Geometry: final body of the model. Coordinates: model frame, mm. Give positions to 0.01 mm unless a question says otherwise; leave off trailing zeros. Write each loop counter-clockwise with the first axis right and the second up, starting at its lowest first coordinate (ties: lowest second). Pieces come first, ordered by that corner, then holes. Notation, with made-up numbers: M 44.25,37 L 93.25,37 A37 cw 93.25,74 Z; hole C 33,30.5 d9. An arc over 180 degrees is marked long. Answer as a JSON object with one key per item and string values.
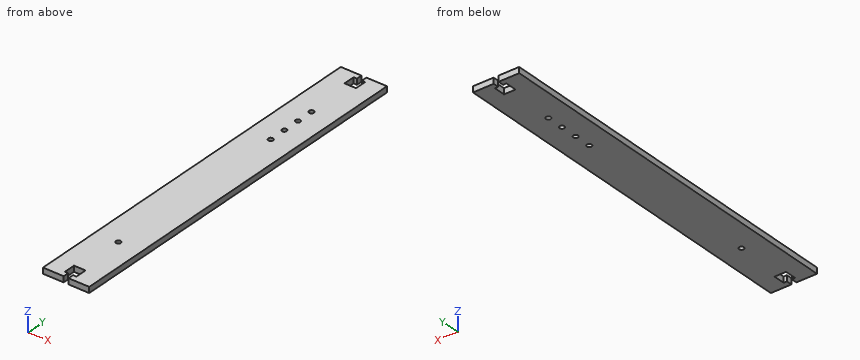
from build123d import *

# Parameters (mm, degrees)
SKETCH1_W           = 40
SKETCH1_H           = 327.5
BOSS_EXTRUDE1_DEPTH = 5
SKETCH2_R           = 2.1
CUT_EXTRUDE1_DEPTH  = 5
CUT_EXTRUDE2_DEPTH  = 5


with BuildPart() as part:
    # Sketch1 → Boss-Extrude1 (new body)
    with BuildSketch(Plane.XY):
        with Locations((-20, 163.75)):
            Rectangle(SKETCH1_W, SKETCH1_H)
    extrude(amount=BOSS_EXTRUDE1_DEPTH)

    # Sketch2 → Cut-Extrude1 (cut)
    with BuildSketch(Plane(origin=(0, 0, 0), x_dir=(-1, 0, 0), z_dir=(0, 0, -1))):
        with Locations((20, 57.5)):
            Circle(SKETCH2_R)
        with Locations((20, 270)):
            Circle(SKETCH2_R)
        with Locations((20, 255)):
            Circle(SKETCH2_R)
        with Locations((20, 240)):
            Circle(SKETCH2_R)
        with Locations((20, 225)):
            Circle(SKETCH2_R)
    extrude(amount=-CUT_EXTRUDE1_DEPTH, mode=Mode.SUBTRACT)

    # Sketch3 → Cut-Extrude2 (cut)
    with BuildSketch(Plane(origin=(0, 0, 0), x_dir=(-1, 0, 0), z_dir=(0, 0, -1))):
        Polygon((17.9, 0), (22.1, 0), (22.1, 5), (25, 5), (25, 15), (15, 15), (15, 5), (17.9, 5), align=None)
    cut_extrude2 = extrude(amount=-CUT_EXTRUDE2_DEPTH, mode=Mode.SUBTRACT)

    # Mirror1: Cut-Extrude2 across plane
    add(cut_extrude2.mirror(Plane.ZX.offset(163.75)), mode=Mode.SUBTRACT)


solid = part.part
1) Line query: line 1 (Y direction, x = -20, z = 1.2); line 2 (Y direction, x = -20.5, z = 4.3); line 3 (X direction, y = 225, z = 1.4). Output: solid intervals per line, ascending. Write a range as from..to.
Geometry check:
{"line 1": "y = 15..55.4, 59.6..222.9, 227.1..237.9, 242.1..252.9, 257.1..267.9, 272.1..312.5", "line 2": "y = 15..55.46, 59.54..222.96, 227.04..237.96, 242.04..252.96, 257.04..267.96, 272.04..312.5", "line 3": "x = -40..-22.1, -17.9..0"}
2) Cut plane A-A on z = 3.7. Return loops of the section in (x, y).
Geometry check:
{"outline": "M -40,0 L -22.1,0 L -22.1,5 L -25,5 L -25,15 L -15,15 L -15,5 L -17.9,5 L -17.9,0 L 0,0 L 0,327.5 L -17.9,327.5 L -17.9,322.5 L -15,322.5 L -15,312.5 L -25,312.5 L -25,322.5 L -22.1,322.5 L -22.1,327.5 L -40,327.5 Z; hole C -20,57.5 d4.2; hole C -20,225 d4.2; hole C -20,240 d4.2; hole C -20,255 d4.2; hole C -20,270 d4.2"}
3) Contact query for a flat-ended pin moving along its axis: P1, Ø2.5, axis at x = -19.5, z = 2.5, coming from the +Y side. Output: stop coordinate, or through.
Geometry check:
{"P1": "stops at y = 312.5"}
